Can you work these out from the drawing? Everything is in mm from the part's minimum corner. A direction names the side the tool comes from. Give positions to 0.01 mm unless a question says otherwise; leave off trailing zeros. Write each loop counter-clockwise with the first axis right and the second up, starting at its lowest first coordinate (ties: lowest second). Pieces come first, ordered by that corner, then holes. Notation, with made-up numbers: (58.25, 57.25) - (63.25, 57.25) arc R18 cw to (63.25, 86.25) - close; hole circle Ø7 at (-11.75, -14.75). An arc over 180 degrees is marked (long way). Write each question's results on one line, items separated by ' | '. Start each with the question number.
Item 1: Suppose I cut it at C-C on y = 7.25. List the corners of the cut face in (x, z) for me, then the cut area to 3 significant figures.
Item 2: Will these pins go through, and if not, where does the flat tip stop? P1, Ø4, axis at x = 45.5, y = 7.5, coming from the +Z side; P2, Ø4.5, axis at x = 35, z = 106.84, coming from the +Y side; P3, Ø4, axis at x = 24, z = 85, coming from the +Y side; P4, Ø3, axis at y = 3.5, z = 99, coming from the -X side.
Item 3: Please list where these lines run through material, in increasing order: line 1 along Z through (x, y) = (52.5, 7.25); line 2 along Z through (x, y) = (30.5, 1.75).
Item 4: Which directions (+Z, -Z, +X, -X, +Y, -Y) give clear straight access to the entire face, cutting with the end or side of a thin tool? Please do the marked faces 3, 4 and 5.
Item 5: We'd pull the mould along X, two halves only. Please class the marked faces 1 and 2: +X half, -X half, draft (parallel to the pull), parting line (faces both ways), or undercut.
Item 6: Suppose I cut it at D-D on z = 71.5. List the corners of the cut face in (x, y) for me.
Item 7: Suppose I cut it at A-A on x = 40.5. List the corners of the cut face in (y, z) for me.
Item 8: Suppose I cut it at B-B on z = 52. List the corners of the cut face in (x, y) for me.
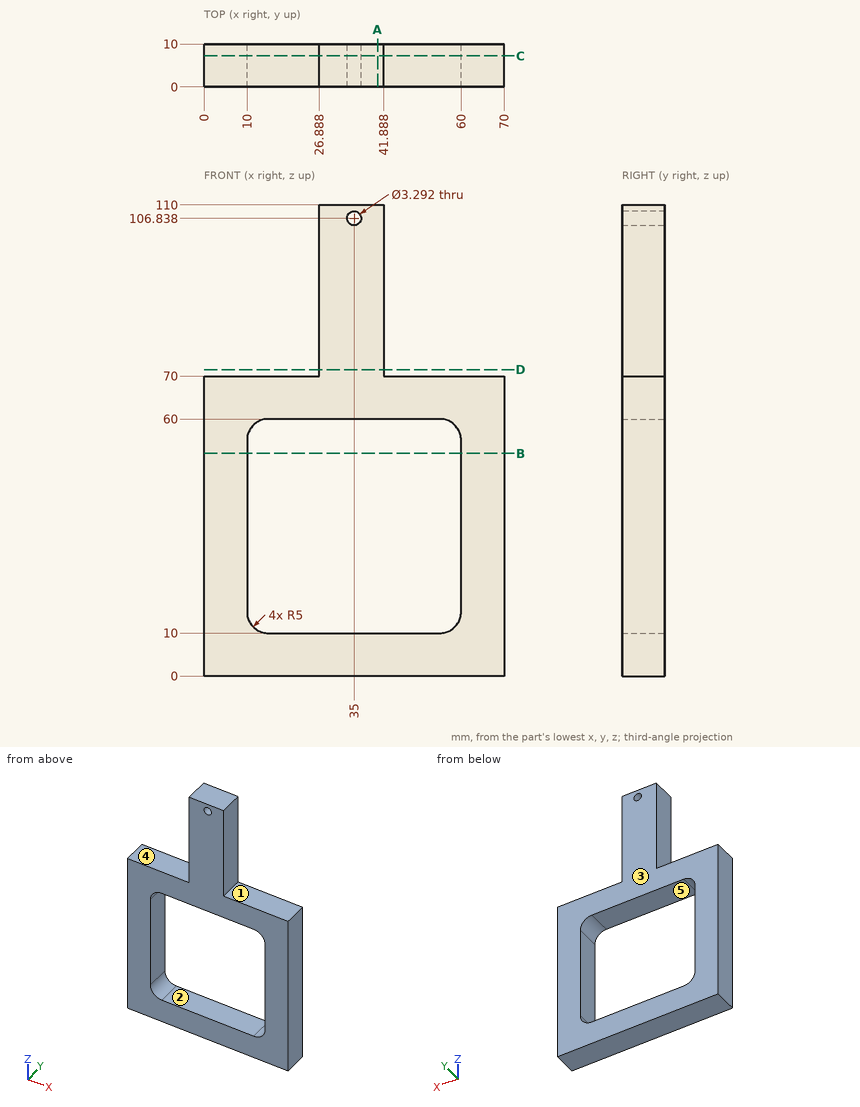
Checked values:
1) outline: (0, 0) - (70, 0) - (70, 70) - (41.89, 70) - (41.89, 110) - (26.89, 110) - (26.89, 70) - (0, 70) - close; hole (10, 15) arc R5 ccw to (15, 10) - (55, 10) arc R5 ccw to (60, 15) - (60, 55) arc R5 ccw to (55, 60) - (15, 60) arc R5 ccw to (10, 55) - close; hole circle Ø3.29 at (35, 106.84) | area: 3,010 mm^2
2) P1: stops at z = 70 | P2: stops at y = 10 | P3: passes through | P4: stops at x = 26.89
3) line 1: z = 0 to 10, 60 to 70 | line 2: z = 0 to 10, 60 to 110
4) face 3: +Z, -Z, +X, -X, +Y | face 4: +Z, -X, +Y, -Y | face 5: +Y, -Y
5) face 1: draft | face 2: undercut
6) outline: (26.89, 0) - (41.89, 0) - (41.89, 10) - (26.89, 10) - close
7) outline: (0, 0) - (10, 0) - (10, 10) - (0, 10) - close; (0, 60) - (10, 60) - (10, 110) - (0, 110) - close
8) outline: (0, 0) - (10, 0) - (10, 10) - (0, 10) - close; (60, 0) - (70, 0) - (70, 10) - (60, 10) - close
